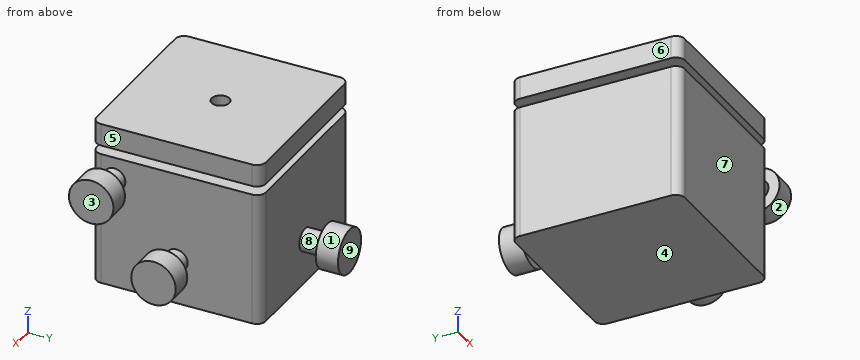
Autodesk Inventor part; units mm, degrees
ref_plane "YZ Plane" through (0, 0, 0) normal (1, 0, 0) x (0, 1, 0)
ref_plane "XZ Plane" through (0, 0, 0) normal (0, 1, 0) x (-1, 0, 0)
ref_plane "XY Plane" through (0, 0, 0) normal (0, 0, 1) x (1, 0, 0)
sketch "Sketch1" plane through (0, 0, 0) normal (0, 0, 1) x (1, 0, 0)
  line L0 (19, -19) -> (-19, -19)
  line L1 (-19, -19) -> (-19, 19)
  line L2 (-19, 19) -> (19, 19)
  line L3 (19, 19) -> (19, -19)
  line L4 (19, -19) -> (-19, 19) construction
  line L5 (-19, -19) -> (19, 19) construction
  point P0 (0, 0)
  dimension "d0" = 38
  dimension "d1" = 38
extrude "Extrusion1" add sketch "Sketch1" along normal blind 30
sketch "Sketch2" plane through (0, 0, 30) normal (0, 0, 1) x (1, 0, 0)
  circle A0 centre (0, 0) radius 2.5
  dimension "d4" = 5
extrude "Extrusion2" add sketch "Sketch2" along normal blind 2
sketch "Sketch3" plane through (0, 0, 32) normal (0, 0, 1) x (1, 0, 0)
  line L0 (19, 19) -> (-19, 19)
  line L1 (-19, 19) -> (-19, -19)
  line L2 (-19, -19) -> (19, -19)
  line L3 (19, -19) -> (19, 19)
  point P0 (0, 0)
extrude "Extrusion3" add sketch "Sketch3" along normal blind 5
sketch "Sketch4" plane through (-19, 19, 0) normal (0, 1, 0) x (1, 0, 0)
  circle A0 centre (19, -10) radius 2.5
  point P0 (19, 0)
  dimension "d9" = 5
extrude "Extrusion4" add sketch "Sketch4" along normal blind 5
sketch "Sketch5" plane through (0, 24, 10) normal (0, 1, 0) x (1, 0, 0)
  circle A0 centre (0, 0) radius 5
  point P0 (0, 10)
  dimension "d12" = 10
extrude "Extrusion5" add sketch "Sketch5" along normal blind 5
sketch "Sketch6" plane through (19, -19, 0) normal (1, 0, 0) x (0, 0, -1)
  circle A0 centre (-10, 19) radius 2.5
  circle A1 centre (-25, 5) radius 2.5
  point P0 (0, 19)
  dimension "d15" = 5
  dimension "d16" = 5
extrude "Extrusion6" add sketch "Sketch6" along normal blind 5
sketch "Sketch7" plane through (24, 0, 10) normal (1, 0, 0) x (0, 0, -1)
  circle A0 centre (0, 0) radius 5
  circle A1 centre (-15, -14) radius 2.5
  circle A2 centre (-15, -14) radius 5
  point P0 (10, 0)
  dimension "d19" = 10
  dimension "d20" = 10
extrude "Extrusion7" add sketch "Sketch7" along normal blind 5 contours A0 | A1 | A2
fillet "Fillet1" radius 2 8 edges at (19, 19, 15) (19, 19, 34.5) (19, -19, 15) (-19, 19, 15) (19, -19, 34.5) (-19, -19, 15) (-19, -19, 34.5) (-19, 19, 34.5)
sketch "Sketch8" plane through (0, 0, 37) normal (0, 0, 1) x (1, 0, 0)
  circle A0 centre (0, 0) radius 2
  dimension "d24" = 4
extrude "Extrusion8" cut sketch "Sketch8" against normal blind 5
properties part number "RadiantDyes-RD-PDT-S(appox)"
Could you check a few things on this model? Use its own coordinates, in mm. Face numbers are marked on the shaded views. A direction names the side the tool comes from. Round coordinates to 2 decimals unless told otherwise and drop trailing zeros. Loops run counter-clockwise (first coordinate to the right, second up) from the corner with the lowest first, then second, coordinate; pieces in that order, holes last. Notation, with made-up numbers: (36.5, -32.5) - (89.5, -32.5) arc R19 ccw to (89.5, -1.5) - close; hole circle Ø10 at (-25, -22). An arc over 180 degrees is marked (long way). Answer as CSV lines item,"result".
1. I want a section at A-A on y = -14. List the corners of the cut face in (x, z) for me, then the cut area to 4 significant figures.
Filled in:
outline,"(-19, 0) - (19, 0) - (19, 22.5) - (24, 22.5) - (24, 20) - (29, 20) - (29, 30) - (24, 30) - (24, 27.5) - (19, 27.5) - (19, 30) - (-19, 30) - close; (-19, 32) - (19, 32) - (19, 37) - (-19, 37) - close"
area,"1,405 mm^2"
2. I want a section at C-C on z = 25. List the corners of the cut face in (x, y) for me.
Filled in:
outline,"(-19, -17) arc R2 ccw to (-17, -19) - (17, -19) arc R2 ccw to (19, -17) - (19, -16.5) - (24, -16.5) - (24, -19) - (29, -19) - (29, -9) - (24, -9) - (24, -11.5) - (19, -11.5) - (19, 17) arc R2 ccw to (17, 19) - (-17, 19) arc R2 ccw to (-19, 17) - close"
3. For pin 1 Ø3 at (x, z) = (16.5, 16.5) entering from +Y; pin 2 Ø3.5 at (x, y) = (0, 0) entering from -Z; pin 3 Ø1.5 at (y, z) = (8, 33.5) entering from +X, each with a flat end and sliding along its axis, tell me the tip position at first contact or that it passes through.
Filled in:
pin 1,"stops at y = 19"
pin 2,"stops at z = 0"
pin 3,"stops at x = 19"
4. I want a section at B-B on x = -9.5. List the corners of the cut face in (y, z) for me, then the cut area to 3 significant figures.
Filled in:
outline,"(-19, 0) - (19, 0) - (19, 30) - (-19, 30) - close; (-19, 32) - (19, 32) - (19, 37) - (-19, 37) - close"
area,"1,330 mm^2"
5. We'd pull the mould along Y, two halves only. Please class the marked faces 6, 7, 8 and 9: +Y half, -Y half, draft (parallel to the pull), parting line (faces both ways), or undercut.
Filled in:
face 6,"draft"
face 7,"-Y half"
face 8,"undercut"
face 9,"+Y half"
6. I want a section at D-D on y = 0. List the corners of the cut face in (x, z) for me, then the cut area to 4 significant figures.
Filled in:
outline,"(-19, 0) - (19, 0) - (19, 7.5) - (24, 7.5) - (24, 5) - (29, 5) - (29, 15) - (24, 15) - (24, 12.5) - (19, 12.5) - (19, 30) - (2.5, 30) - (2.5, 32) - (19, 32) - (19, 37) - (2, 37) - (2, 32) - (-2, 32) - (-2, 37) - (-19, 37) - (-19, 32) - (-2.5, 32) - (-2.5, 30) - (-19, 30) - close"
area,"1,395 mm^2"
7. Please list where these lines run through material, in increasing order: line 1 along Z through (x, y) = (18, 16.5); line 2 along Y through (x, z) = (0, 35.15); line 3 along X through (y, z) = (2, 8). Write a range as [from, to].
Filled in:
line 1,"z = [0, 30], [32, 37]"
line 2,"y = [-19, -2], [2, 19]"
line 3,"x = [-19, 19], [24, 29]"
8. On a 3-axis mill with a long thin cutter (end or side, diameter ignored), from which of +Z, -Z, +X, -X, +Y, -Y can I reach the whole of each face in a straight line? I mean the marked faces 1, 2, 3, 4 and 5. Say none if no direction works.
Filled in:
face 1,"+Y"
face 2,"+X"
face 3,"+Z, -Z, +X, +Y, -Y"
face 4,"-Z, +X, -X, +Y, -Y"
face 5,"+Z, +X, +Y, -Y"
